Here's how the part is built. I have some questions about the finished solid (model axes, mm). Face numbers are marked on the shaded views. Round coordinates to 2 decimals unless told otherwise and drop trailing zeros. Order: outer loops, then holes, each group sorted by start corner. A loop starts at its lowest first (then second) coordinate and runs counter-clockwise, first axis right, second up. Notation, with made-up numbers: (79, 25) - (95, 25) arc R35 ccw to (95, 61) - close; hole circle Ø3 at (32, 19). An arc over 180 degrees is marked (long way). Answer as a JSON object with one key per item and string values.
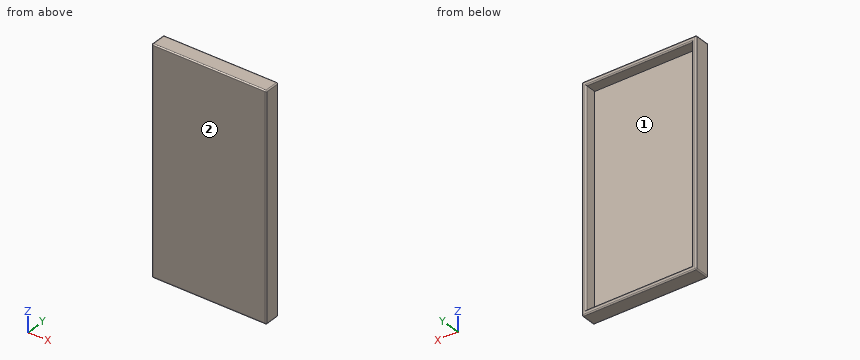
Autodesk Fusion 360 part; units mm, degrees
sketch "Sketch1" plane through (0, 0, 0) normal (0, 1, 0) x (1, 0, 0)
  line L0 (0, 0) -> (23.5, 0)
  line L1 (23.5, 0) -> (23.5, 47.5)
  line L2 (23.5, 47.5) -> (0, 47.5)
  line L3 (0, 47.5) -> (0, 0)
  line L4 (-1, -1) -> (24.5, -1)
  line L5 (24.5, -1) -> (24.5, 48.5)
  line L6 (24.5, 48.5) -> (-1, 48.5)
  line L7 (-1, 48.5) -> (-1, -1)
  dimension "d1" = 23.5
  dimension "d2" = 47.5
  dimension "d3" = 1
extrude "Extrude1" add sketch "Sketch1" along normal blind 1 contours L0 L1 L2 L3
extrude "Extrude2" add sketch "Sketch1" along normal blind 3.5
fillet "Fillet1" radius 0.25 7 edges at (11.75, 0, 1) (24.5, 0, -23.75) (11.75, 3.5, 1) (0, 3.5, -23.75) (11.75, 3.5, -47.5) (23.5, 3.5, -23.75) (11.75, 3.5, 0) 4 faces at (24.5, 1.1667, -15.5) (16, 1.1667, -48.5) (7.5, 0, -32) (-1, 1.1667, -32)
1. Imagine slicing it at B-B (z = -40). List the corners of the cut face in (x, y) for me, plus the area to 3 significant figures.
Responses:
{"outline": "(-1, 0.25) arc R0.25 ccw to (-0.75, 0) - (24.25, 0) arc R0.25 ccw to (24.5, 0.25) - (24.5, 3.25) arc R0.25 ccw to (24.25, 3.5) - (23.75, 3.5) arc R0.25 ccw to (23.5, 3.25) - (23.5, 1) - (0, 1) - (0, 3.25) arc R0.25 ccw to (-0.25, 3.5) - (-0.75, 3.5) arc R0.25 ccw to (-1, 3.25) - close", "area": "30.4 mm2"}
2. Imagine slicing it at A-A (y = 2). List the corners of the cut face in (x, z) for me, plus the area to 3 significant figures.
Responses:
{"outline": "(-1, -48.25) arc R0.25 ccw to (-0.75, -48.5) - (24.25, -48.5) arc R0.25 ccw to (24.5, -48.25) - (24.5, 0.75) arc R0.25 ccw to (24.25, 1) - (-0.75, 1) arc R0.25 ccw to (-1, 0.75) - close; hole (0, -47.5) - (23.5, -47.5) - (23.5, 0) - (0, 0) - close", "area": "146 mm2"}
3. If I drill on L1, parallel to X at y = 1.6, z = -39; L2, parallel to Z at x = 20.25, y = 2.9; L3, parallel to Y at x = 6.25, z = -42, over which ranges is the centre line in solid material (lowest first)? Write a range as [from, to].
Responses:
{"L1": "[-1, 0], [23.5, 24.5]", "L2": "[-48.5, -47.5], [0, 1]", "L3": "[0, 1]"}
4. Imagine slicing it at C-C (x = 11.25). List the corners of the cut face in (y, z) for me.
Responses:
{"outline": "(0, -48.25) arc R0.25 ccw to (0.25, -48.5) - (3.25, -48.5) arc R0.25 ccw to (3.5, -48.25) - (3.5, -47.75) arc R0.25 ccw to (3.25, -47.5) - (1, -47.5) - (1, 0) - (3.25, 0) arc R0.25 ccw to (3.5, 0.25) - (3.5, 0.75) arc R0.25 ccw to (3.25, 1) - (0.25, 1) arc R0.25 ccw to (0, 0.75) - close"}
5. For P1, Ø7, axis at x = 14.5, z = -17, coming from the +Y side, with a flat end and sliding along its axis, tell me the tip position at first contact or that it passes through.
Responses:
{"P1": "y = 1"}
6. Thinking about a two-plate mould opening in X: for the marked faces 1 and 2, which applies, pulls with the +X half, pulls with the -X half, needs draft (parallel to the pull), parting line crosses it, or undercut?
Responses:
{"face 1": "undercut", "face 2": "needs draft"}
